Could you check a few things on this drawing? It's one solid part, dimensions in mm from its lowest x, y, z. Give positions to 0.01 mm unless a question says otherwise; leave off trailing zeros. Loops run counter-clockwise (first coordinate to the right, second up) from the corner with the lowest first, then second, coordinate; pieces in that order, holes last. Notation, with made-up numbers: (50, 8.25) - (76, 8.25) arc R30 ccw to (76, 32.25) - close; hole circle Ø7 at (-23, -30). An arc over 180 degrees is marked (long way). Return JSON: item names as keys, results as strings. Group by question number.
(1) I need wall thicknesses on probe 1 along X at (y, z) = (1.8, 22.5); probe 2 along Z at (x, y) = (1.75, 1.4) (1 decimal); probe 3 along Z at (x, y) = (18.75, 0.9) (1 decimal). Which ranges of each line are inside material? Lowest first, please. Write a range as [from, to].
(2) If we section it at D-D (y = 0.35): State how many separate pieces and enclosed holes the cut face has, then the cut area to 3 significant figures.
(3) For P1, Ø2.5, axis at x = 5.78, z = 5.78, coming from the +Y side; P2, Ø5, axis at x = 11, z = 16.5, coming from the +Y side; P3, Ø0.6, axis at y = 1, z = 21.5, coming from the +X side (1 decimal); P4, Ø1, axis at y = 1.5, z = 10, coming from the +X side, each with a flat end and sliding along its axis, tell me the tip position at first contact or that it passes through.
(4) If we section it at B-B (x = 22.5): Please give me the cut outline in (y, z).
(5) If we section it at C-C (z = 2.5): Please give me the cut outline in (x, y), then the cut area to 3 significant figures.
(6) If we mould it in two halves opening along Z, with no side actions, what happens to the marked faces 1, 2 and 3? For each: released by +Z, released by -Z, zero draft, split by the parting line, or undercut.
(7) If we section it at A-A (z = 12.5): Please give me the cut outline in (x, y), then the cut area to 3 significant figures.
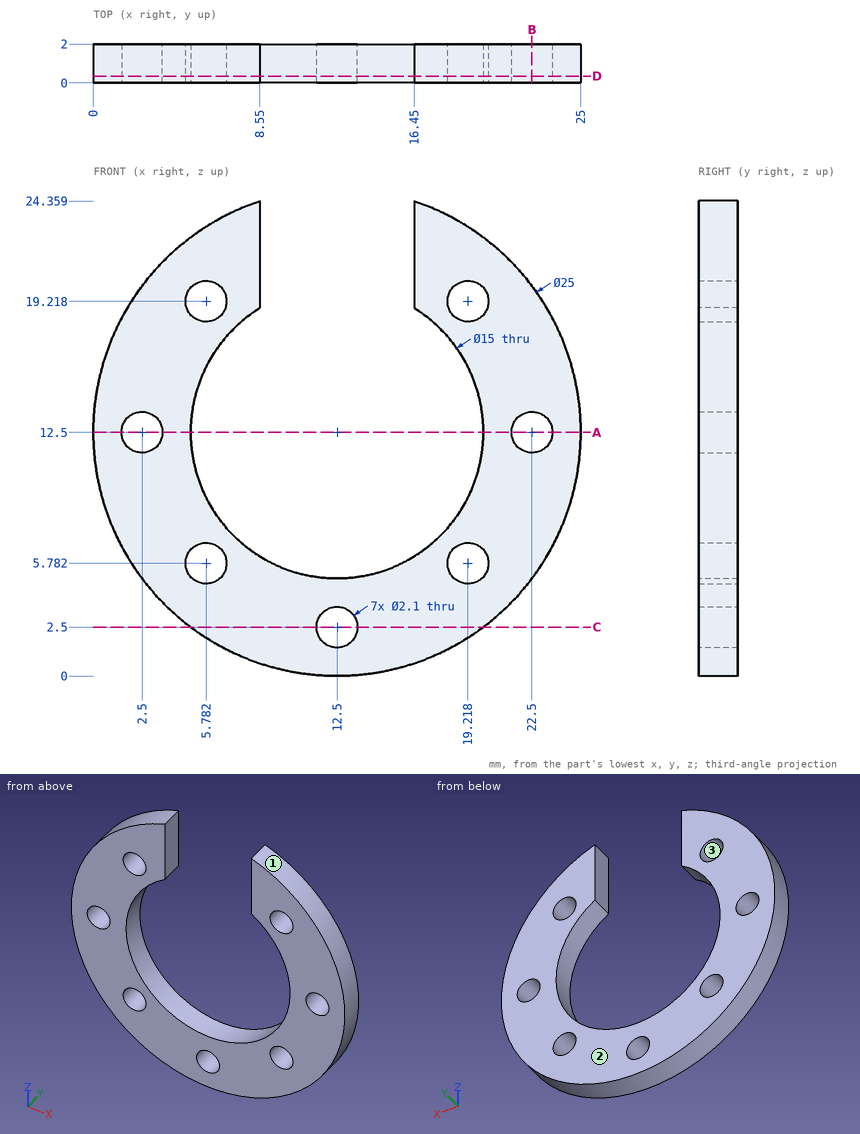
Values:
{
 "1": {"probe 1": "[5, 8.55], [16.45, 20]", "probe 2": "[6.1, 11.8], [13.2, 18.9]", "probe 3": "[1.7, 4.8], [6.7, 8.4], [16.6, 18.3], [20.2, 23.3]"},
 "2": {"separate pieces": "1", "enclosed holes": "7", "area": "249 mm2"},
 "3": {"P1": "y = 2", "P2": "through", "P3": "x = 21.5", "P4": "x = 24.84"},
 "4": {"outline": "(0, 5) - (2, 5) - (2, 11.45) - (0, 11.45) - close; (0, 13.55) - (2, 13.55) - (2, 20) - (0, 20) - close"},
 "5": {"outline": "(5, 0) - (11.45, 0) - (11.45, 2) - (5, 2) - close; (13.55, 0) - (20, 0) - (20, 2) - (13.55, 2) - close", "area": "25.8 mm2"},
 "6": {"face 1": "split by the parting line", "face 2": "zero draft", "face 3": "undercut"},
 "7": {"outline": "(0, 0) - (1.45, 0) - (1.45, 2) - (0, 2) - close; (3.55, 0) - (5, 0) - (5, 2) - (3.55, 2) - close; (20, 0) - (21.45, 0) - (21.45, 2) - (20, 2) - close; (23.55, 0) - (25, 0) - (25, 2) - (23.55, 2) - close", "area": "11.6 mm2"}
}
